For this review, use the dimensioned drawing (mm, ordinates from the lowest corner) and the shaded views. A direction names the side the tool comes from. Give positions to 0.01 mm unless a question says otherwise; leave off trailing zeros. Loops run counter-clockwise (first coordinate to the right, second up) from the corner with the lowest first, then second, coordinate; pieces in that order, holes last. Notation, with made-up numbers: (88, -34) - (128, -34) arc R4 cw to (128, -30) - close; hole circle Ø3 at (13, -36). An arc over 180 degrees is marked (long way). Put each result on its own line as item: value.
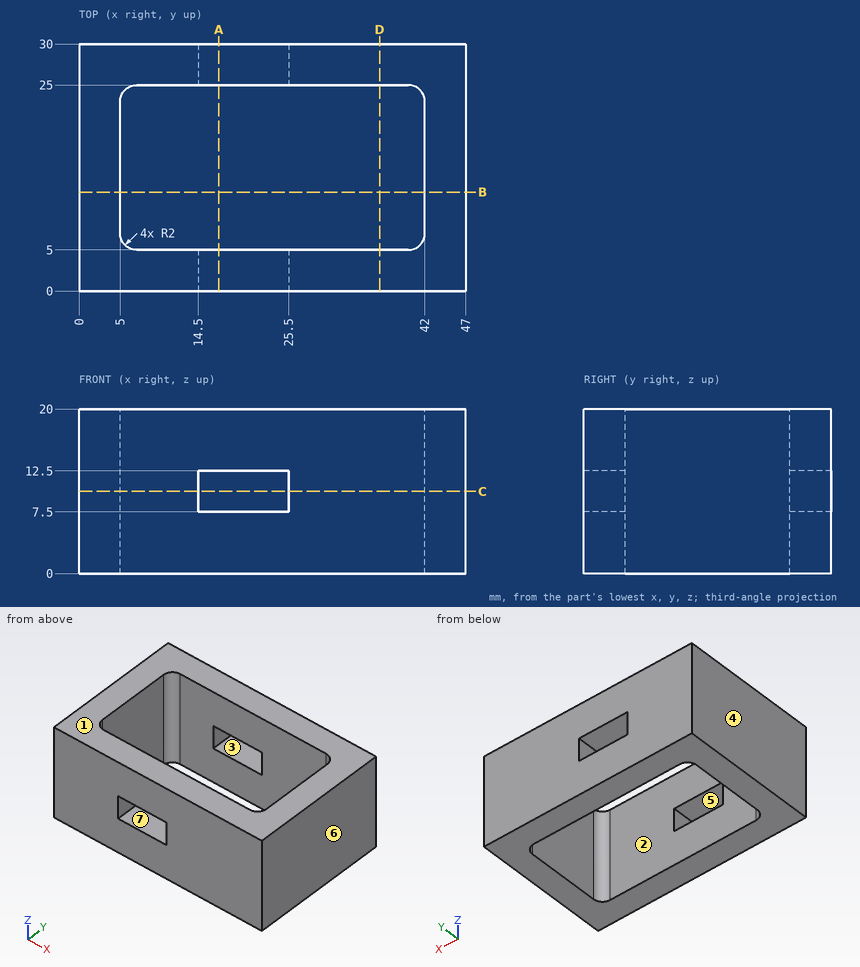
1) Take a section at C-C on z = 10. State the section outline as (x, y) points, and give its area (3 significant figures).
Geometry check:
outline: (0, 0) - (14.5, 0) - (14.5, 5) - (7, 5) arc R2 cw to (5, 7) - (5, 23) arc R2 cw to (7, 25) - (14.5, 25) - (14.5, 30) - (0, 30) - close; (25.5, 0) - (47, 0) - (47, 30) - (25.5, 30) - (25.5, 25) - (40, 25) arc R2 cw to (42, 23) - (42, 7) arc R2 cw to (40, 5) - (25.5, 5) - close
area: 563 mm²
2) Insertion check: pin 1 Ø2.5 at (x, y) = (22.5, 26.5) entering from -Z. The pin has a flat end and moves straight along its axis. Give the tip position at first contact, or say it passes through.
Geometry check:
pin 1: stops at z = 0
3) Wall thickness on line 1 (Y direction, x = 36, z = 13); line 2 (Z direction, x = 23.5, y = 27); line 3 (X direction, y = 9, z = 18): over which ranges is each line inside the solid? List them lowest first.
Geometry check:
line 1: y = 0 to 5, 25 to 30
line 2: z = 0 to 7.5, 12.5 to 20
line 3: x = 0 to 5, 42 to 47
4) Draft analysis for pull direction X (two halves, no side actions). For the marked faces 4, 5, 6 and 7, state which applies: pulls with the +X half, pulls with the -X half, needs draft (parallel to the pull), parting line crosses it, or undercut.
Geometry check:
face 4: pulls with the -X half
face 5: undercut
face 6: pulls with the +X half
face 7: undercut
5) Take a section at B-B on y = 12. State the section outline as (x, z) points.
Geometry check:
outline: (0, 0) - (5, 0) - (5, 20) - (0, 20) - close; (42, 0) - (47, 0) - (47, 20) - (42, 20) - close
6) For the marked faces 1, 2 and 3, list the 3-axis set-ups (+Z, -Z, +X, -X, +Y, -Y) from which the entire face can be reached by the end or side of a thin tool; tool diameter is ignored.
Geometry check:
face 1: +Z, +X, -X, +Y, -Y
face 2: +Z, -Z
face 3: +Y, -Y
7) Take a section at A-A on x = 17. State the section outline as (y, z) points, and give its area (3 significant figures).
Geometry check:
outline: (0, 0) - (5, 0) - (5, 7.5) - (0, 7.5) - close; (0, 12.5) - (5, 12.5) - (5, 20) - (0, 20) - close; (25, 0) - (30, 0) - (30, 7.5) - (25, 7.5) - close; (25, 12.5) - (30, 12.5) - (30, 20) - (25, 20) - close
area: 150 mm²
8) Take a section at D-D on x = 36.5. State the section outline as (y, z) points.
Geometry check:
outline: (0, 0) - (5, 0) - (5, 20) - (0, 20) - close; (25, 0) - (30, 0) - (30, 20) - (25, 20) - close
